The figure shows three views and two pictorial views of one solid part (mm, origin at its lowest corner). Answer the questions. A direction names the side the tool comes from. Coordinates: 2 decimals unless noted, no trailing zeros. Write each loop counter-clockwise with the first axis right and the second up, starting at its lowest first coordinate (ties: lowest second). Pieces come first, ordered by that corner, then holes.
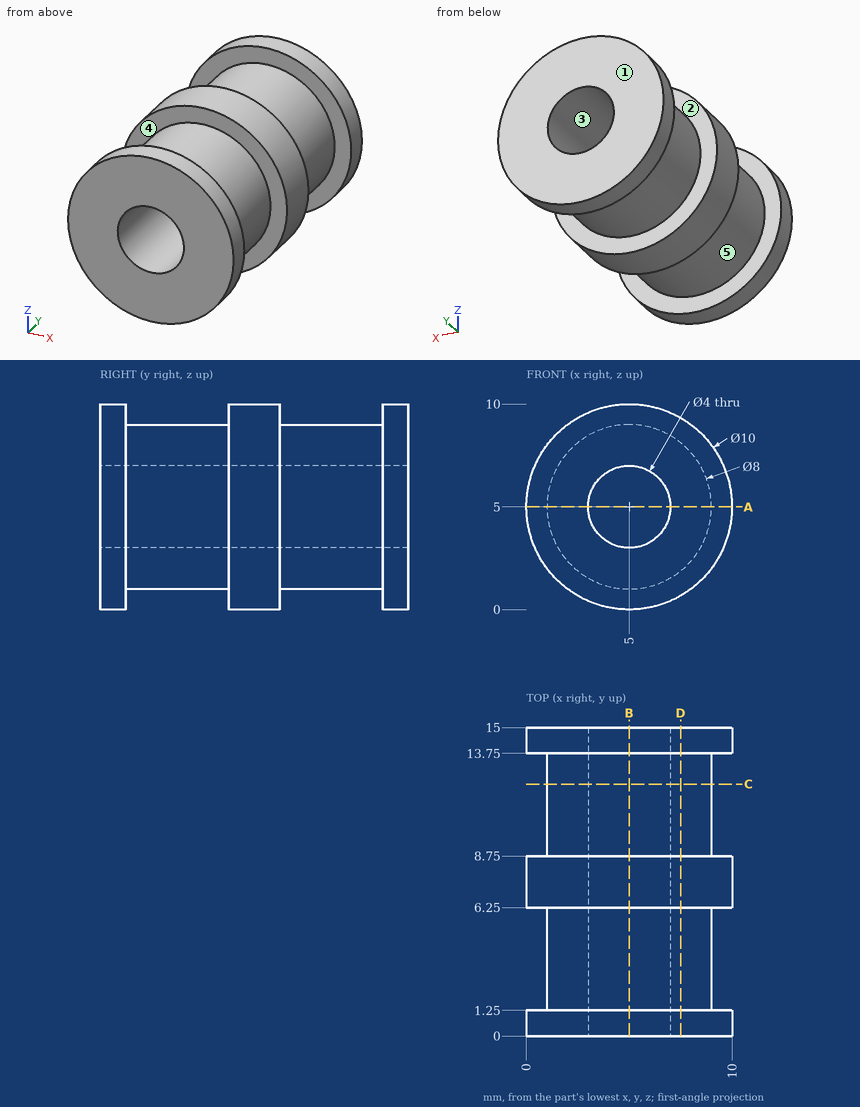
Item 1: The part is cut by section A-A (z = 5). Give the vertices of the cut face in (x, y).
Item 2: The part is cut by section C-C (y = 12.25). Give the vertices of the cut face in (x, z).
Item 3: Find the intervals of material crossed by probe 1 along Y at (x, z) = (1.75, 8.25); probe 2 along X at (y, z) = (9.75, 5); probe 3 along X at (y, z) = (6.75, 5), in increasing order.
Item 4: Determine the mould class of the marked faces 3, 4 and 5 for opening direction Z: +Z half, -Z half, draft (parallel to the pull), parting line (faces both ways), or undercut.
Item 5: The part is cut by section D-D (x = 7.5). Give the vertices of the cut face in (y, z).
Item 6: The part is cut by section B-B (x = 5). Give the vertices of the cut face in (y, z), and give its area (3 significant figures).
Item 7: For the marked faces 1 and 2, determine the directions among +Z, -Z, +X, -X, +Y, -Y from which every point of the face is accessible in a straight line to the end or side of a thin tool.
Item 8: Given pin 1 (2.5 mm diameter, centred on x = 5, z = 5, fed in from +Y); pin 2 (5 mm diameter, centred on y = 8, z = 9, fed in from -X); pin 3 (1.5 mm diameter, centred on y = 7, z = 8.5, fed in from -X); pin 4 (2 mm diameter, centred on x = 7, y = 5, fed in from +Z), each flat-ended and moving along its own axis, determine where each tip first touches the part or whether it passes through.
Answer:
1. outline: (0, 0) - (3, 0) - (3, 15) - (0, 15) - (0, 13.75) - (1, 13.75) - (1, 8.75) - (0, 8.75) - (0, 6.25) - (1, 6.25) - (1, 1.25) - (0, 1.25) - close; (7, 0) - (10, 0) - (10, 1.25) - (9, 1.25) - (9, 6.25) - (10, 6.25) - (10, 8.75) - (9, 8.75) - (9, 13.75) - (10, 13.75) - (10, 15) - (7, 15) - close
2. outline: circle Ø8 at (5, 5); hole circle Ø4 at (5, 5)
3. probe 1: y = 0 to 1.25, 6.25 to 8.75, 13.75 to 15
3. probe 2: x = 1 to 3, 7 to 9
3. probe 3: x = 0 to 3, 7 to 10
4. face 3: undercut
4. face 4: draft
4. face 5: parting line
5. outline: (0, 0.67) - (1.25, 0.67) - (1.25, 1.88) - (6.25, 1.88) - (6.25, 0.67) - (8.75, 0.67) - (8.75, 1.88) - (13.75, 1.88) - (13.75, 0.67) - (15, 0.67) - (15, 9.33) - (13.75, 9.33) - (13.75, 8.12) - (8.75, 8.12) - (8.75, 9.33) - (6.25, 9.33) - (6.25, 8.12) - (1.25, 8.12) - (1.25, 9.33) - (0, 9.33) - close
6. outline: (0, 0) - (1.25, 0) - (1.25, 1) - (6.25, 1) - (6.25, 0) - (8.75, 0) - (8.75, 1) - (13.75, 1) - (13.75, 0) - (15, 0) - (15, 3) - (0, 3) - close; (0, 7) - (15, 7) - (15, 10) - (13.75, 10) - (13.75, 9) - (8.75, 9) - (8.75, 10) - (6.25, 10) - (6.25, 9) - (1.25, 9) - (1.25, 10) - (0, 10) - close
6. area: 70.0 mm2
7. face 1: +Z, -Z, +X, -X, +Y
7. face 2: none
8. pin 1: passes through
8. pin 2: stops at x = 0.23
8. pin 3: stops at x = 0.82
8. pin 4: stops at z = 8.87
